Build history of the part. All positions in model axes, mm. Face numbers are marked on the shaded views. A direction names the side the tool comes from. Coordinates: 2 decimals unless noted, no trailing zeros. Loops run counter-clockwise (first coordinate to the right, second up) from the corner with the lowest first, then second, coordinate; pieces in that order, holes last. Notation, with made-up numbers: (48.5, -27) - (86.5, -27) arc R22 ccw to (86.5, -18) - close; hole circle Ø1 at (77.5, 40). An arc over 180 degrees is marked (long way). One line per item, written item: value.
```python
from build123d import *

# Parameters (mm, degrees)
SKETCH2_W           = 40
SKETCH2_H           = 30
BOSS_EXTRUDE1_DEPTH = 10
SKETCH3_R           = 1.55
CUT_EXTRUDE1_DEPTH  = 4
SKETCH4_R           = 4.8125
CUT_EXTRUDE2_DEPTH  = 4
SKETCH7_R           = 3.325
CUT_EXTRUDE3_DEPTH  = 1


with BuildPart() as part:
    # Sketch2 → Boss-Extrude1 (new body)
    with BuildSketch(Plane(origin=(0, 0, 0), x_dir=(1, 0, 0), z_dir=(0, 1, 0))):
        Rectangle(SKETCH2_W, SKETCH2_H)
    extrude(amount=BOSS_EXTRUDE1_DEPTH)

    # Sketch3 → Cut-Extrude1 (cut)
    with BuildSketch(Plane(origin=(0, 0, 0), x_dir=(-1, 0, 0), z_dir=(0, -1, 0))):
        with Locations(Location((-13.333333333, -10, 0), (0, 0, 90))):
            Circle(SKETCH3_R)
        with Locations(Location((13.333333333, -10, 0), (0, 0, 270))):
            Circle(SKETCH3_R)
        with Locations(Location((-13.333333333, 10, 0), (0, 0, 270))):
            Circle(SKETCH3_R)
        with Locations(Location((13.333333333, 10, 0), (0, 0, 90))):
            Circle(SKETCH3_R)
    extrude(amount=-CUT_EXTRUDE1_DEPTH, mode=Mode.SUBTRACT)

    # Sketch4 → Cut-Extrude2 (cut)
    with BuildSketch(Plane(origin=(0, 10, 0), x_dir=(1, 0, 0), z_dir=(0, 1, 0))):
        with Locations(Location((7.9286, -6.465, 0), (0, 0, 270))):
            Circle(SKETCH4_R)
        with Locations(Location((-7.5, 6.4636, 0), (0, 0, 270))):
            Circle(SKETCH4_R)
    extrude(amount=-CUT_EXTRUDE2_DEPTH, mode=Mode.SUBTRACT)

    # Sketch7 → Cut-Extrude3 (cut)
    with BuildSketch(Plane(origin=(0, 6, 0), x_dir=(1, 0, 0), z_dir=(0, 1, 0))):
        with Locations(Location((7.9286, -6.465, 0), (0, 0, 270))):
            Circle(SKETCH7_R)
        with Locations(Location((-7.5, 6.4636, 0), (0, 0, 270))):
            Circle(SKETCH7_R)
    extrude(amount=-CUT_EXTRUDE3_DEPTH, mode=Mode.SUBTRACT)


solid = part.part
```
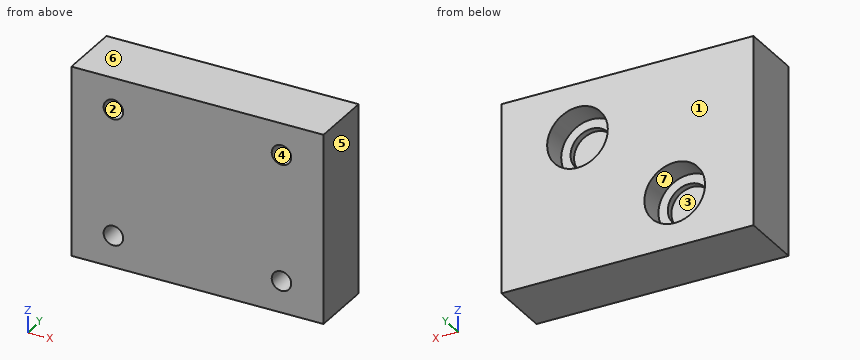
Item 1: Probe probe 1 along X at (y, z) = (2.7, -10); probe 2 along Y at (x, z) = (-9, -7.5); probe 3 along X at (y, z) = (6.25, -7.5). List the from-to ranges inside material, lowest first. Write a range as from..to.
Check result:
probe 1: x = -20..-14.88, -11.78..11.78, 14.88..20
probe 2: y = 0..5
probe 3: x = -20..-12.2, -2.8..20
Item 2: Cut at C-C, the plane y = 1.5. Write the cut outline in (x, z).
Check result:
outline: (-20, -15) - (20, -15) - (20, 15) - (-20, 15) - close; hole circle Ø3.1 at (-13.33, -10); hole circle Ø3.1 at (-13.33, 10); hole circle Ø3.1 at (13.33, -10); hole circle Ø3.1 at (13.33, 10)
Item 3: Pull direction Z, two halves, no side cores. Call the marked faces 4, 5, 6 and 7: released by +Z, released by -Z, zero draft, split by the parting line, or undercut.
Check result:
face 4: undercut
face 5: zero draft
face 6: released by +Z
face 7: undercut
Item 4: Cut at D-D, the plane y = 7. Write the cut outline in (x, z) (1 decimal).
Check result:
outline: (-20, -15) - (20, -15) - (20, 15) - (-20, 15) - close; hole circle Ø9.6 at (-7.5, -6.5); hole circle Ø9.6 at (7.9, 6.5)
Item 5: Drop flat-ended pins along their axis: P1, Ø0.9, axis at x = -12.5, z = -10, coming from the -Y side; P2, Ø3.5, axis at x = -6.5, z = -6, coming from the +Y side; P3, Ø8.5, axis at x = 7.93, z = 6.46, coming from the +Y side. Give the stop position or say it passes through.
Check result:
P1: stops at y = 4
P2: stops at y = 5
P3: stops at y = 6
Item 6: Cut at B-B, the plane z = 9. Write the cut outline in (x, y).
Check result:
outline: (-20, 0) - (-14.52, 0) - (-14.52, 4) - (-12.15, 4) - (-12.15, 0) - (12.15, 0) - (12.15, 4) - (14.52, 4) - (14.52, 0) - (20, 0) - (20, 10) - (12.02, 10) - (12.02, 6) - (10.08, 6) - (10.08, 5) - (5.78, 5) - (5.78, 6) - (3.84, 6) - (3.84, 10) - (-20, 10) - close
Item 7: Tool access for the marked faces 1, 2 and 3: list every direction of +Z, -Z, +X, -X, +Y, -Y with a clear straight run to the whole face (end or side of a thin tool).
Check result:
face 1: +Z, -Z, +X, -X, +Y
face 2: -Y
face 3: +Y
Item 8: Cut at A-A, the plane x = -7.5. Write the cut outline in (y, z).
Check result:
outline: (0, -15) - (10, -15) - (10, -11.28) - (6, -11.28) - (6, -9.79) - (5, -9.79) - (5, -3.14) - (6, -3.14) - (6, -1.65) - (10, -1.65) - (10, 15) - (0, 15) - close
